```python
from build123d import *

# Parameters (mm, degrees)
SKETCH1_R           = 3.175
BOSS_EXTRUDE1_DEPTH = 10
FILLET1_R           = 3


with BuildPart() as part:
    # Sketch1 → Boss-Extrude1 (new body)
    with BuildSketch(Plane.XY):
        with BuildLine():
            Line((1.941142838, 7.244443697), (-22.207002819, 13.714919825))
            Line((-22.207002819, 13.714919825), (-26.089288495, -0.77396757))
            Line((-26.089288495, -0.77396757), (-3.871447622, -6.727220089))
            Line((-3.871447622, -6.727220089), (6.671220145, -23))
            Line((6.671220145, -23), (10.921738991, -18.749481154))
            Line((10.921738991, -18.749481154), (7.386058148, 1.302361333))
            ThreePointArc((7.386058148, 1.302361333), (5.529580026, 5.066926557), (1.941142838, 7.244443697))
        make_face()
        Circle(SKETCH1_R, mode=Mode.SUBTRACT)
    extrude(amount=BOSS_EXTRUDE1_DEPTH)

    # Fillet1
    fillet1_edges = [part.edges().sort_by_distance(p)[0] for p in [
        (-3.871447622, -6.727220089, 5),
        (-26.089288495, -0.77396757, 5),
        (-22.207002819, 13.714919825, 5),
    ]]
    fillet(fillet1_edges, radius=FILLET1_R)


solid = part.part
```
Geometry check sheet. Reference: the model listing, model coordinates, mm. Round coordinates to 2 decimals unless told otherwise and drop trailing zeros. Loops run counter-clockwise (first coordinate to the right, second up) from the corner with the lowest first, then second, coordinate; pieces in that order, holes last. Notation, with made-up numbers: (-38.75, 42) -> (-0.75, 42) arc R27 cw to (-0.75, 72) -> close; hole circle Ø6 at (61, 86.5). An arc over 180 degrees is marked (long way). Use a Markdown table: item, result.
(1) Go/stop test with flat-tipped pins: P1, Ø5, axis at y = 8.5, z = 4.5, coming from the +X side; P2, Ø5, axis at x = -6, z = 6.5, coming from the -Y side; P3, Ø1.5, axis at y = -3.5, z = 6, coming from the +X side. Record where each tip stops, or that it passes through.
Calculated:
| item | result |
|---|---|
| P1 | x = 4.5 |
| P2 | y = -7.36 |
| P3 | x = 8.37 |
(2) Sectioned sample at C-C (y = 0). Enter the section's corners in (x, z) (3 decimals).
Calculated:
| item | result |
|---|---|
| outline | (-25.095, 0) -> (-3.175, 0) -> (-3.175, 10) -> (-25.095, 10) -> close; (3.175, 0) -> (7.616, 0) -> (7.616, 10) -> (3.175, 10) -> close |
(3) Mould release check, pull along X, two halves, no side actions. Record for faces 1 (the flat face through (9.179, -8.864, 4.93)), 2 (the cylindrical face through (-4, -6.9, 5.1)), 3 (the cylindrical face through (-21.557, 12.655, 5.07)), 4 (the cylindrical face through (-0.69, -3.1, 4.93)): released by +X, released by -X, zero draft, split by the parting line, or undercut.
Calculated:
| item | result |
|---|---|
| face 1 | released by +X |
| face 2 | released by -X |
| face 3 | split by the parting line |
| face 4 | undercut |
(4) Scan lines: probe 1 along Y at (x, z) = (0, 7.75) (3 decimals); probe 2 along X at (y, z) = (2, 6.25); probe 3 along Y at (x, z) = (2, 2.5). Record each from-to range of solid material in increasing order.
Calculated:
| item | result |
|---|---|
| probe 1 | -12.703 to -3.175, 3.175 to 7.765 |
| probe 2 | -25.34 to -2.47, 2.47 to 7.23 |
| probe 3 | -15.79 to -2.47, 2.47 to 7.23 |
(5) Sectioned sample at D-D (y = -11). Enter the section's corners in (x, z).
Calculated:
| item | result |
|---|---|
| outline | (-1.1, 0) -> (9.56, 0) -> (9.56, 10) -> (-1.1, 10) -> close |
(6) Sectioned sample at B-B (x = -0.5). Enter the section's corners in (y, z), then the cut area to 3 significant figures.
Calculated:
| item | result |
|---|---|
| outline | (-11.93, 0) -> (-3.14, 0) -> (-3.14, 10) -> (-11.93, 10) -> close; (3.14, 0) -> (7.9, 0) -> (7.9, 10) -> (3.14, 10) -> close |
| area | 136 mm² |
(7) Sectioned sample at A-A (z = 5.5). Enter the section's corners in (x, y) (3 decimals), then the cut area to 3 significant figures.
Calculated:
| item | result |
|---|---|
| outline | (-25.313, 2.124) arc R3 ccw to (-23.192, -1.55) -> (-4.986, -6.429) arc R3 cw to (-3.244, -7.695) -> (6.671, -23) -> (10.922, -18.749) -> (7.386, 1.302) arc R7.5 ccw to (1.941, 7.244) -> (-19.309, 12.938) arc R3 ccw to (-22.983, 10.817) -> close; hole circle Ø6.35 at (0, 0) |
| area | 570 mm² |
